Build history of the part. All positions in model axes, mm. Face numbers are marked on the shaded views. A direction names the side the tool comes from. Give positions to 0.01 mm unless a question says otherwise; leave off trailing zeros. Order: outer loops, then holes, each group sorted by start corner. A loop starts at its lowest first (then second) coordinate and runs counter-clockwise, first axis right, second up. Notation, with made-up numbers: (-38, 10) - (-9, 10) arc R33 ccw to (-9, 46) - close; hole circle Ø5 at (18.5, 37). An arc over 180 degrees is marked (long way). Use a Markdown table: item, result. Add a question column.
(1) Slice it at C-C (x = 0). Write the cut outline in (y, z), then the cut area to 3 significant figures.
(2) Slice it at D-D (y = -23). Write the cut outline in (x, z), then the cut area to 3 significant figures.
(3) Flat gauge pins, fed straight in: pin 1 (14 mm diameter, centred on y = -18, z = 24, fed in from -X); pin 2 (7.5 mm diameter, centred on x = -20.5, y = -16, fed in from +Z); pin 3 (4 mm diameter, centred on y = -16, z = 20.5, fed in from +X). Where does each tip first touch, or does it go through?
(4) Slice it at A-A (y = -15.25). Write the cut outline in (x, z).
(5) Which spindle directions (+Z, -Z, +X, -X, +Y, -Y) get a long thin tool onto all of the face, cutting with end or side? Do the marked faces 4 and 5. Say none if no direction does.
(6) Wall check: line 1 (Z direction, x = 32, y = -7.5); line 2 (X direction, y = -8.25, z = 18); line 3 (X direction, y = -18.75, z = 24.5). Give the ranges that are in metal, low to high.
(7) Mould opens along X. For the marked faces 1, 2 and 3 say: +X half, -X half, draft (parallel to the pull), parting line (faces both ways), or undercut.
from build123d import *

# Parameters (mm, degrees)
F1_DEPTH = 25.4
F2_R     = 6.35
F3_DEPTH = 25.4
F4_R     = 6.35
F5_DEPTH = 25.4
F6_R     = 6.35
F7_DEPTH = 25.4


with BuildPart() as f1:
    # F0 (on Front) → F1 (new body)
    with BuildSketch(Plane.XZ):
        Polygon((-13.694073, 16.45344), (-39.094073, 16.45344), (-39.094073, 3.75344), (37.105927, 3.75344), (37.105927, 16.45344), (11.705927, 16.45344), (11.705927, 41.85344), (-13.694073, 41.85344), align=None)
    extrude(amount=F1_DEPTH)

    # F2 (on face) → F3 (cut)
    with BuildSketch(Plane.XZ.offset(25.4)):
        with Locations((-0.994073, 29.15344)):
            Circle(F2_R)
        with BuildLine():
            ThreePointArc((-13.694073, 29.15344), (-9.974329, 38.133696), (-0.994073, 41.85344))
            Line((-0.994073, 41.85344), (-13.694073, 41.85344))
            Line((-13.694073, 41.85344), (-13.694073, 29.15344))
        make_face()
        with BuildLine():
            ThreePointArc((-0.994073, 41.85344), (7.986183, 38.133696), (11.705927, 29.15344))
            Line((11.705927, 29.15344), (11.705927, 41.85344))
            Line((11.705927, 41.85344), (-0.994073, 41.85344))
        make_face()
    extrude(amount=-F3_DEPTH, mode=Mode.SUBTRACT)

    # F4 (on face) → F5 (cut)
    with BuildSketch(Plane.XY.offset(16.45344)):
        with Locations((-26.394073, -12.7)):
            Circle(F4_R)
        with BuildLine():
            ThreePointArc((-26.394073, -25.4), (-38.757753, -12.7), (-26.394073, 0))
            Line((-26.394073, 0), (-39.094073, 0))
            Line((-39.094073, 0), (-39.094073, -25.4))
            Line((-39.094073, -25.4), (-26.394073, -25.4))
        make_face()
    extrude(amount=-F5_DEPTH, mode=Mode.SUBTRACT)

    # F6 (on face) → F7 (cut)
    with BuildSketch(Plane.XY.offset(16.45344)):
        with Locations((24.405927, -12.7)):
            Circle(F6_R)
        with BuildLine():
            ThreePointArc((24.405927, 0), (33.386183, -3.719744), (37.105927, -12.7))
            Line((37.105927, -12.7), (37.105927, 0))
            Line((37.105927, 0), (24.405927, 0))
        make_face()
        with BuildLine():
            ThreePointArc((37.105927, -12.7), (33.386183, -21.680256), (24.405927, -25.4))
            Line((24.405927, -25.4), (37.105927, -25.4))
            Line((37.105927, -25.4), (37.105927, -12.7))
        make_face()
    extrude(amount=-F7_DEPTH, mode=Mode.SUBTRACT)


solid = f1.part
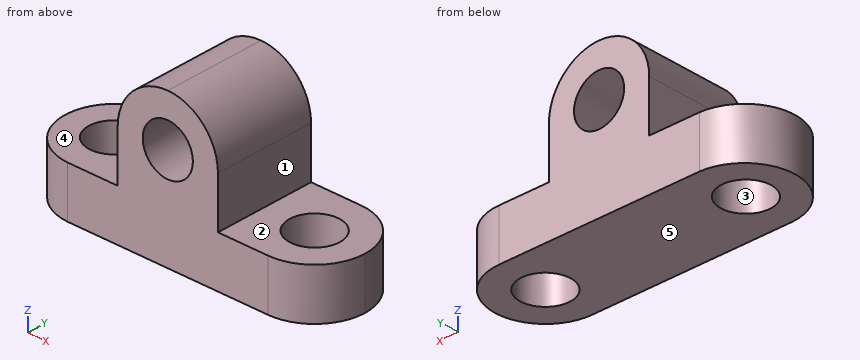
Solution:
| question | item | result |
|---|---|---|
| 1 | outline | (-25.4, 3.75) - (0, 3.75) - (0, 22.88) - (-25.4, 22.88) - close; (-25.4, 35.43) - (0, 35.43) - (0, 41.81) - (-25.4, 41.81) - close |
| 1 | area | 648 mm2 |
| 2 | outline | (-33.49, 3.75) - (31.84, 3.75) - (31.84, 16.45) - (11.71, 16.45) - (11.71, 29.15) arc R12.7 ccw to (-13.69, 29.15) - (-13.69, 16.45) - (-33.49, 16.45) - close; hole circle Ø12.7 at (-0.99, 29.15) |
| 2 | area | 1,280 mm2 |
| 3 | pin 1 | x = -13.69 |
| 3 | pin 2 | z = 16.45 |
| 3 | pin 3 | x = 11.71 |
| 4 | outline | (-38.5, 3.75) - (-32.21, 3.75) - (-32.21, 16.45) - (-38.5, 16.45) - close; (-20.58, 3.75) - (18.59, 3.75) - (18.59, 16.45) - (11.71, 16.45) - (11.71, 29.15) arc R12.7 ccw to (-13.69, 29.15) - (-13.69, 16.45) - (-20.58, 16.45) - close; (30.22, 3.75) - (36.85, 3.75) - (36.85, 16.45) - (30.22, 16.45) - close; hole circle Ø12.7 at (-0.99, 29.15) |
| 5 | face 4 | +Z, -X, +Y, -Y |
| 5 | face 5 | -Z, +X, -X, +Y, -Y |
| 6 | line 1 | 3.75 to 16.45 |
| 6 | line 2 | -13.69 to 11.71 |
| 6 | line 3 | -13.69 to -5.31, 3.33 to 11.71 |
| 7 | face 1 | +X half |
| 7 | face 2 | draft |
| 7 | face 3 | undercut |
